```python
from build123d import *

# Parameters (mm, degrees)
F2_SIZE  = 3
F3_R     = 2.5
F4_W     = 4
F4_H     = 1.5
F5_DEPTH = 20
F6_SIZE  = 1
F7_SIZE  = 2
F8_SIZE  = 1


with BuildPart() as f1:
    # F0 (on Front) → F1 (revolve)
    with BuildSketch(Plane.XZ):
        Polygon((-32.5, 0), (-23.5, 0), (-23.5, 30), (-26, 30), (-26, 10), (-32.5, 10), align=None)
    revolve(axis=Axis((0, 0, 27.1835356757), (0, 0, 1)))

    # F2
    f2_edges = [f1.edges().sort_by_distance(p)[0] for p in [
        (23.5, 0, 0),
    ]]
    chamfer(f2_edges, length=F2_SIZE)

    # F3
    f3_edges = [f1.edges().sort_by_distance(p)[0] for p in [
        (23.5, 0, 3),
    ]]
    fillet(f3_edges, radius=F3_R)

    # F4 (on face) → F5 (join, through all)
    with BuildSketch(Plane.XY.offset(30)):
        with Locations((0, -26.25)):
            Rectangle(F4_W, F4_H)
        Polygon((22.3826859022, -15.2320508076), (24.3826859022, -11.7679491924), (23.0836477965, -11.0179491924), (21.0836477965, -14.4820508076), align=None)
        Polygon((24.3826859022, 11.7679491924), (22.3826859022, 15.2320508076), (21.0836477965, 14.4820508076), (23.0836477965, 11.0179491924), align=None)
        with Locations((0, 26.25)):
            Rectangle(F4_W, F4_H)
        Polygon((-22.3826859022, 15.2320508076), (-24.3826859022, 11.7679491924), (-23.0836477965, 11.0179491924), (-21.0836477965, 14.4820508076), align=None)
        Polygon((-24.3826859022, -11.7679491924), (-22.3826859022, -15.2320508076), (-21.0836477965, -14.4820508076), (-23.0836477965, -11.0179491924), align=None)
    extrude(amount=-F5_DEPTH)

    # F6
    f6_edges = [f1.edges().sort_by_distance(p)[0] for p in [
        (-26, 0, 30),
        (-13, 22.51666, 30),
        (13, 22.51666, 30),
        (26, 0, 30),
        (13, -22.51666, 30),
        (-13, -22.51666, 30),
    ]]
    chamfer(f6_edges, length=F6_SIZE)

    # F7
    f7_edges = [f1.edges().sort_by_distance(p)[0] for p in [
        (23.382686, -13.5, 30),
        (23.382686, 13.5, 30),
        (0, 27, 30),
        (-23.382686, 13.5, 30),
        (-23.382686, -13.5, 30),
        (0, -27, 30),
    ]]
    chamfer(f7_edges, length=F7_SIZE)

    # F8
    f8_edges = [f1.edges().sort_by_distance(p)[0] for p in [
        (32.5, 0, 0),
    ]]
    chamfer(f8_edges, length=F8_SIZE)


solid = f1.part
```
Read the model definition and answer for the solid it produces. Units are mm, in the model's axes. A direction names the side the tool comes from. Give positions to 0.01 mm unless a question says otherwise; leave off trailing zeros. Write each loop counter-clockwise with the first axis right and the second up, starting at its lowest first coordinate (ties: lowest second). Pieces come first, ordered by that corner, then holes. Notation, with made-up numbers: M 11.25,-25.5 L 60.25,-25.5 A23 cw 60.25,13.5 Z; hole C 48.25,-19.5 d7. An arc over 180 degrees is marked long. Put each result on its own line as item: value. Start each with the question number.
1. Which of the six approach directions +Z, -Z, +X, -X, +Y, -Y give full straight-line access (tool end or side, diameter ignored) to faces 1 (the flat face through (-21.87, 14.936, 20.14)), 2 (the flat face through (-23.895, 11.486, 20.14)), 3 (the flat face through (-23.37, 13.52, 19.13)), 4 (the flat face through (2, 26.4, 20.1)), 5 (the flat face through (23.37, -13.52, 19.13))?
2. Consider line 1 along Y through (x, z) = (0, 22); line 2 along X through (y, z) = (0, 22.25); line 3 along X through (y, z) = (15, 15). Determine where each line is inside the solid, lowest interval first.
3. For a pull along Y with two mould halves and no side action, classify faces 6 (the cylindrical face through (-22.4, -7.1, 17.2)), 7 (the flat face through (0, 26, 29)), 8 (the flat face through (-17, -17, 30)) as released by +Y, released by -Y, zero draft, split by the parting line, or undercut.
4. Each of these flat-tipped pins is pushed along its axis until it touches: pin 1 Ø3 at (x, z) = (-1, 18.5) entering from -Y; pin 2 Ø19.5 at (x, y) = (1.5, 8.5) entering from +Z; pin 3 Ø2 at (x, z) = (0.5, 23.5) entering from +Y; pin 4 Ø12 at (x, z) = (20.5, 19.5) entering from +Y. Where does it stop, or does it pass through?
5. The part is cut by section A-A, the plane z = 12.5. Give the vertices of the cut face in (x, y).
Final values:
1. face 1: +Z, +Y
1. face 2: +Z, -X
1. face 3: +Z, -X, +Y
1. face 4: +Z, +X, +Y
1. face 5: +Z, +X, -Y
2. line 1: y = -27 to -23.5, 23.5 to 27
2. line 2: x = -26 to -23.5, 23.5 to 26
2. line 3: x = -22.52 to -21.98, -21.24 to -18.09, 18.09 to 21.24, 21.98 to 22.52
3. face 6: undercut
3. face 7: released by +Y
3. face 8: zero draft
4. pin 1: stops at y = -27
4. pin 2: passes through
4. pin 3: stops at y = 27
4. pin 4: stops at y = 21.58
5. outline: M -24.38,-11.77 L -22.38,-15.23 L -21.45,-14.69 A26 ccw -2,-25.92 L -2,-27 L 2,-27 L 2,-25.92 A26 ccw 21.45,-14.69 L 22.38,-15.23 L 24.38,-11.77 L 23.45,-11.23 A26 ccw 23.45,11.23 L 24.38,11.77 L 22.38,15.23 L 21.45,14.69 A26 ccw 2,25.92 L 2,27 L -2,27 L -2,25.92 A26 ccw -21.45,14.69 L -22.38,15.23 L -24.38,11.77 L -23.45,11.23 A26 ccw -23.45,-11.23 Z; hole C 0,0 d47
